Autodesk Inventor part; units mm, degrees
ref_plane "YZ Plane" through (0, 0, 0) normal (1, 0, 0) x (0, 1, 0)
ref_plane "XZ Plane" through (0, 0, 0) normal (0, 1, 0) x (-1, 0, 0)
ref_plane "XY Plane" through (0, 0, 0) normal (0, 0, 1) x (1, 0, 0)
sketch "Esboço1" plane through (0, 0, 0) normal (0, 0, 1) x (1, 0, 0)
  line L0 (60, -135) -> (-60, -135)
  line L1 (-60, -135) -> (-60, 135)
  line L2 (-60, 135) -> (60, 135)
  line L3 (60, 135) -> (60, -135)
  line L4 (60, -135) -> (-60, 135) construction
  line L5 (-60, -135) -> (60, 135) construction
  line L6 (-60, 135) -> (60, 135)
  line L7 (60, 135) -> (60, 165)
  line L8 (60, 165) -> (-60, 165)
  line L9 (-60, 165) -> (-60, 135)
  line L10 (60, 165) -> (100, 165)
  line L11 (100, 165) -> (60, 135)
  point P0 (0, 0)
  dimension "d0" = 120
  dimension "d1" = 270
  dimension "d2" = 120
  dimension "d3" = 30
  dimension "d4" = 40
extrude "Extrusão1" add sketch "Esboço1" along normal blind 3
sketch "Esboço2" plane through (60, -135, 0) normal (1, 0, 0) x (0, 0, -1)
  line L0 (-3, 0) -> (0, 0)
  line L1 (0, 0) -> (0, 15)
  line L2 (0, 15) -> (-3, 15)
  line L3 (-3, 15) -> (-3, 0)
  line L4 (-3, 30) -> (0, 30)
  line L5 (0, 30) -> (0, 45)
  line L6 (0, 45) -> (-3, 45)
  line L7 (-3, 45) -> (-3, 30)
  line L8 (-3, 60) -> (0, 60)
  line L9 (0, 60) -> (0, 75)
  line L10 (0, 75) -> (-3, 75)
  line L11 (-3, 75) -> (-3, 60)
  line L12 (-3, 90) -> (0, 90)
  line L13 (0, 90) -> (0, 105)
  line L14 (0, 105) -> (-3, 105)
  line L15 (-3, 105) -> (-3, 90)
  line L16 (-3, 120) -> (0, 120)
  line L17 (0, 120) -> (0, 135)
  line L18 (0, 135) -> (-3, 135)
  line L19 (-3, 135) -> (-3, 120)
  line L20 (-3, 150) -> (0, 150)
  line L21 (0, 150) -> (0, 165)
  line L22 (0, 165) -> (-3, 165)
  line L23 (-3, 165) -> (-3, 150)
  line L24 (-3, 180) -> (0, 180)
  line L25 (0, 180) -> (0, 195)
  line L26 (0, 195) -> (-3, 195)
  line L27 (-3, 195) -> (-3, 180)
  line L28 (-3, 210) -> (0, 210)
  line L29 (0, 210) -> (0, 225)
  line L30 (0, 225) -> (-3, 225)
  line L31 (-3, 225) -> (-3, 210)
  line L32 (-3, 240) -> (0, 240)
  line L33 (0, 240) -> (0, 255)
  line L34 (0, 255) -> (-3, 255)
  line L35 (-3, 255) -> (-3, 240)
  dimension "d7" = 3
  dimension "d8" = 15
  dimension "d11" = 30
sketch "Esboço3" plane through (-60, -135, 0) normal (0, -1, 0) x (1, 0, 0)
  line L0 (160, 3) -> (0, 3)
  line L1 (0, 0) -> (15, 0)
  line L2 (15, 0) -> (15, 3)
  line L3 (15, 3) -> (0, 3)
  line L4 (0, 3) -> (0, 0)
  line L5 (30, 0) -> (45, 0)
  line L6 (45, 0) -> (45, 3)
  line L7 (45, 3) -> (30, 3)
  line L8 (60, 0) -> (75, 0)
  line L9 (75, 0) -> (75, 3)
  line L10 (75, 3) -> (60, 3)
  line L11 (90, 0) -> (105, 0)
  line L12 (105, 0) -> (105, 3)
  line L13 (105, 3) -> (90, 3)
  line L14 (30, 0) -> (45, 0)
  line L15 (45, 3) -> (30, 3)
  line L16 (45, 0) -> (45, 3)
  line L17 (30, 3) -> (30, 0)
  line L18 (60, 0) -> (75, 0)
  line L19 (75, 3) -> (60, 3)
  line L20 (75, 0) -> (75, 3)
  line L21 (60, 3) -> (60, 0)
  line L22 (90, 0) -> (105, 0)
  line L23 (105, 3) -> (90, 3)
  line L24 (105, 0) -> (105, 3)
  line L25 (90, 3) -> (90, 0)
  dimension "d16" = 15
  dimension "d17" = 3
  dimension "d20" = 30
  dimension "d27" = 30
sketch "Esboço4" plane through (-60, 165, 0) normal (0, 1, 0) x (1, 0, 0)
  line L0 (160, -3) -> (0, -3)
  line L1 (0, -3) -> (15, -3)
  line L2 (15, -3) -> (15, 0)
  line L3 (15, 0) -> (0, 0)
  line L4 (0, 0) -> (0, -3)
  line L5 (30, -3) -> (45, -3)
  line L6 (45, -3) -> (45, 0)
  line L7 (45, 0) -> (30, 0)
  line L8 (30, 0) -> (30, -3)
  line L9 (60, -3) -> (75, -3)
  line L10 (75, -3) -> (75, 0)
  line L11 (75, 0) -> (60, 0)
  line L12 (60, 0) -> (60, -3)
  line L13 (90, -3) -> (105, -3)
  line L14 (105, -3) -> (105, 0)
  line L15 (105, 0) -> (90, 0)
  line L16 (90, 0) -> (90, -3)
  line L17 (120, -3) -> (135, -3)
  line L18 (135, -3) -> (135, 0)
  line L19 (135, 0) -> (120, 0)
  line L20 (120, 0) -> (120, -3)
  point P0 (15, -3)
  dimension "d32" = 15
  dimension "d33" = 3
  dimension "d43" = 30
sketch "Esboço5" plane through (100, 165, 0) normal (0.6, -0.8, 0) x (0.8, 0.6, 0)
  line L0 (0, 0) -> (-128, 0)
  line L1 (0, 0) -> (-10, 0)
  line L2 (-50, 0) -> (0, 0)
  line L3 (-10, 0) -> (-40, 0)
  line L4 (-40, 0) -> (-40, 3)
  line L5 (-40, 3) -> (-10, 3)
  line L6 (-10, 3) -> (-10, 0)
  point P0 (-179, 0)
  point P1 (-40, 0)
  dimension "d34" = 10
  dimension "d35" = 30
  dimension "d36" = 3
extrude "Extrusão2" add sketch "Esboço2" along normal blind 3
extrude "Extrusão3" add sketch "Esboço3" along normal blind 3
extrude "Extrusão4" add sketch "Esboço4" along normal blind 3
extrude "Extrusão5" add sketch "Esboço5" along normal blind 3
equation "\"d16\" = d8"
equation "\"d17\" = d7"
equation "\"d32\" = d16"
equation "\"d33\" = d17"
equation "\"d36\" = d33"
properties part number "side"
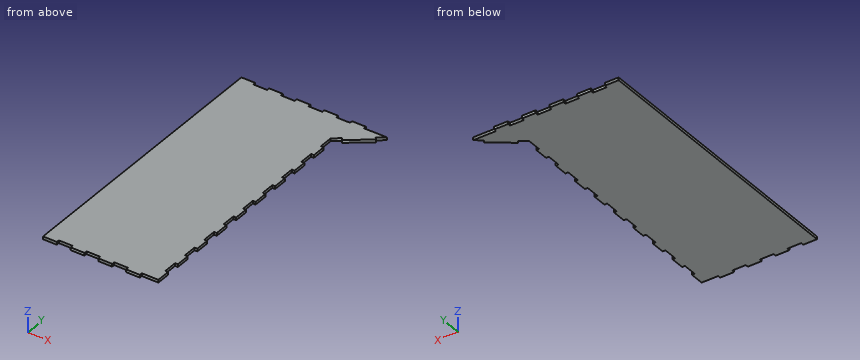
For this review, take the finished solid that the model builds, in its own axes (mm). Give positions to 0.01 mm unless a question says otherwise; leave off trailing zeros. Loops run counter-clockwise (first coordinate to the right, second up) from the corner with the lowest first, then second, coordinate; pieces in that order, holes last. Notation, with made-up numbers: M 81,82 L 99,82 A22 cw 99,93 Z; hole C 3.25,12 d9. An arc over 180 degrees is marked long. Put each result on its own line as item: value. Start each with the question number.
(1) Wall thickness on L1, parallel to Y at x = 46.5, z = 0.7; L2, parallel to X at y = 17.5, z = 2.45; L3, parallel to X at y = 37.5, z = 2.2: over which ranges is each line inside the solid? List them lowest first.
(2) Add section A-A, the plane y = -4. Write out the cut boundary in (x, z), then the cut area to 3 significant figures.
(3) Add section B-B, the plane x = -38. Write out the cut boundary in (y, z), then the cut area to 3 significant figures.
(4) For pin 1 (1.5 mm diameter, centred on y = -37.5, z = 1.5, fed in from +X); pin 2 (0.9 mm diameter, centred on y = -116, z = 2, fed in from +X); pin 3 (1.5 mm diameter, centred on x = -8.5, z = 1.5, fed in from +Y), all flat-tipped, find the tip position at first contact; note any pin that passes through.
Result:
1. L1: y = -135 to 165
1. L2: x = -60 to 63
1. L3: x = -60 to 60
2. outline: M -60,0 L 63,0 L 63,3 L -60,3 Z
2. area: 369 mm^2
3. outline: M -135,0 L 165,0 L 165,3 L -135,3 Z
3. area: 900 mm^2
4. pin 1: stops at x = 63
4. pin 2: stops at x = 60
4. pin 3: stops at y = 165
